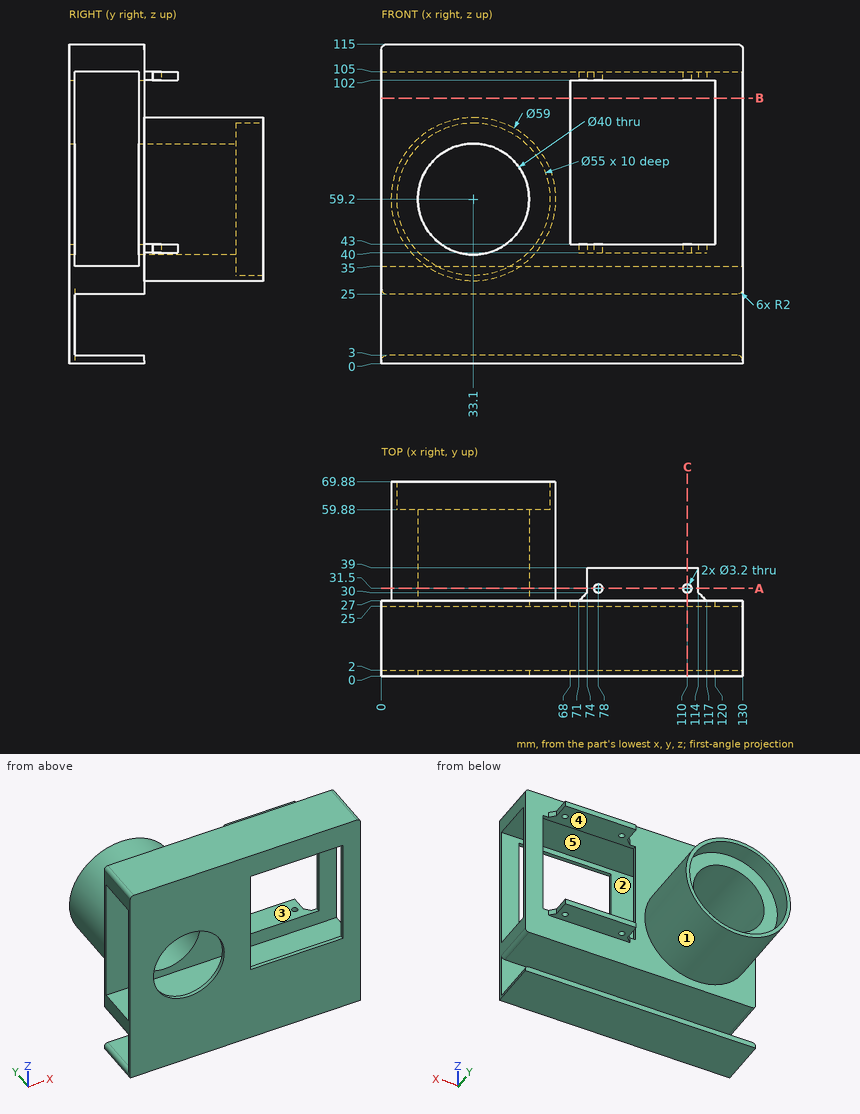
Check sheet for the drawn part. Datum: minimum x, y, z corner. Units: mm. A direction names the side the tool comes from. Give positions to 0.01 mm unless a question says otherwise; leave off trailing zeros. Write each loop counter-clockwise with the first axis right and the second up, starting at its lowest first coordinate (ties: lowest second). Pieces come first, ordered by that corner, then holes. Notation, with made-up numbers: M 10.25,83 L 49.25,83 A18 ccw 49.25,105 Z; hole C 28,-28.5 d8. An arc over 180 degrees is marked long. Write item = value, one per line.
(1) Sectioned sample at A-A (y = 31.5). Record the cut outline in (x, z).
Found:
outline = C 33.1,59.2 d59; M 74,40 L 76.4,40 L 76.4,43 L 74,43 Z; M 74,102 L 76.4,102 L 76.4,105 L 74,105 Z; M 79.6,40 L 108.4,40 L 108.4,43 L 79.6,43 Z; M 79.6,102 L 108.4,102 L 108.4,105 L 79.6,105 Z; M 111.6,40 L 114,40 L 114,43 L 111.6,43 Z; M 111.6,102 L 114,102 L 114,105 L 111.6,105 Z; hole C 33.1,59.2 d40
(2) Access from +Z, -Z, +X, -X, +Y, -Y to the whole of each face (thin tool, end or side, straight path). Record for the marked faces 1, 2 and 3.
Found:
face_1 = +Y
face_2 = +X, -X
face_3 = +Y, -Y
(3) Sectioned sample at B-B (z = 95.5). Record the cut outline in (x, y), then the cut area to 3 significant figures.
Found:
outline = M 0,0 L 68,0 L 68,2 L 0,2 Z; M 0,25 L 68,25 L 68,27 L 0,27 Z; M 120,0 L 130,0 L 130,2 L 120,2 Z; M 120,25 L 130,25 L 130,27 L 120,27 Z
area = 312 mm2
(4) Material ranges on line 1 (Z direction, x = 74, y = 25.5); line 2 (Z direction, x = 55, y = 19.5); line 3 (Z direction, x = 33, y = 52), recorded low to high.
Found:
line_1 = 0 to 3, 25 to 43, 102 to 115
line_2 = 0 to 3, 25 to 35, 105 to 115
line_3 = 29.7 to 39.2, 79.2 to 88.7
(5) Go/stop test with flat-tipped pins: pin 1 Ø7 at (x, y) = (84.5, 29) entering from -Z; pin 2 Ø0.9 at (y, z) = (36.5, 41) entering from -X; pin 3 Ø3.5 at (x, y) = (91, 32) entering from -Z; pin 4 Ø1.5 at (y, z) = (35, 103) entering from +X. Record where each tip stops, or that it passes through.
Found:
pin_1 = 0
pin_2 = 9.54
pin_3 = 40
pin_4 = 114
(6) Draft check along X on the marked faces 4 and 5. Enter one of: released by +X, released by -X, zero draft, split by the parting line, or undercut.
Found:
face_4 = undercut
face_5 = zero draft
(7) Sectioned sample at C-C (x = 110). Give the number of separate pieces and of enclosed holes in the cut face, then the cut area to 3 significant figures.
Found:
separate_pieces = 4
enclosed_holes = 0
area = 762 mm2
